Autodesk Inventor part; units mm, degrees
ref_plane "YZ Plane" through (0, 0, 0) normal (1, 0, 0) x (0, 1, 0)
ref_plane "XZ Plane" through (0, 0, 0) normal (0, 1, 0) x (-1, 0, 0)
ref_plane "XY Plane" through (0, 0, 0) normal (0, 0, 1) x (1, 0, 0)
sketch "Sketch1" plane through (0, 0, 0) normal (0, 0, 1) x (1, 0, 0)
  line L0 (0, 0) -> (150, 0)
  line L1 (150, 0) -> (150, -135)
  line L2 (150, -135) -> (0, -135)
  line L3 (0, -135) -> (0, 0)
  circle A0 centre (3.5, -35) radius 1.5
  line L4 (75, 0) -> (75, -135)
  circle A1 centre (146.5, -35) radius 1.5
  circle A2 centre (3.5, -125) radius 1.5
  circle A3 centre (146.5, -125) radius 1.5
  dimension "d0" = 150
  dimension "d1" = 135
  dimension "d2" = 3
  dimension "d3" = 3.5
  dimension "d4" = 35
  dimension "d5" = 3
  dimension "d6" = 3.5
  dimension "d7" = 90
extrude "Extrusion1" add sketch "Sketch1" along normal blind 7
move faces "Move1" translate (0, -0.3, 0) faces at (100, 0, 2.3333)
move faces "Move2" translate (-0.3, 0, 0) faces at (150, -90.1, 2.3333)
move faces "Move3" translate (0, 0.3, 0) faces at (49.9, -135, 2.3333)
move faces "Move4" translate (0.3, 0, 0) faces at (0, -45.1, 2.3333)
sketch "Sketch3" plane through (0, 0, 0) normal (0, 0, -1) x (-1, 0, 0)
  line L0 (-149.7, -134.7) -> (-149.7, -0.3) construction
  line L1 (-149.7, -23.3) -> (-0.3, -23.3) construction
  line L2 (-0.3, -0.3) -> (-0.3, -134.7) construction
  line L3 (-149.7, -0.3) -> (-0.3, -0.3) construction
  line L4 (-125, -28.3) -> (-25, -28.3)
  line L5 (-25, -28.3) -> (-25, -18.3)
  line L6 (-25, -18.3) -> (-125, -18.3)
  line L7 (-125, -18.3) -> (-125, -28.3)
  line L8 (-125, -28.3) -> (-25, -18.3) construction
  line L9 (-25, -28.3) -> (-125, -18.3) construction
  line L10 (-149.7, -0.3) -> (-0.3, -0.3)
  line L11 (-75, -0.3) -> (-75, -132.391)
  circle A0 centre (-112.5, -69.7) radius 2.5
  line L12 (-0.3, -134.7) -> (-149.7, -134.7)
  circle A1 centre (-37.5, -69.7) radius 2.5
  point P0 (0, 0)
  point P1 (-75, -23.3)
  dimension "d22" = 23
  dimension "d23" = 100
  dimension "d24" = 10
  dimension "d27" = 5
  dimension "d28" = 75
  dimension "d29" = 65
extrude "Extrusion2" cut sketch "Sketch3" against normal through all
sketch "Sketch5" plane through (0, 0, 7) normal (0, 0, 1) x (1, 0, 0)
  point P0 (0, 0)
sketch "Sketch6" plane through (0.3, -134.7, 0) normal (-1, 0, 0) x (0, 0, 1)
  point P0 (0, 134.7)
properties part number "mávač_víčko"
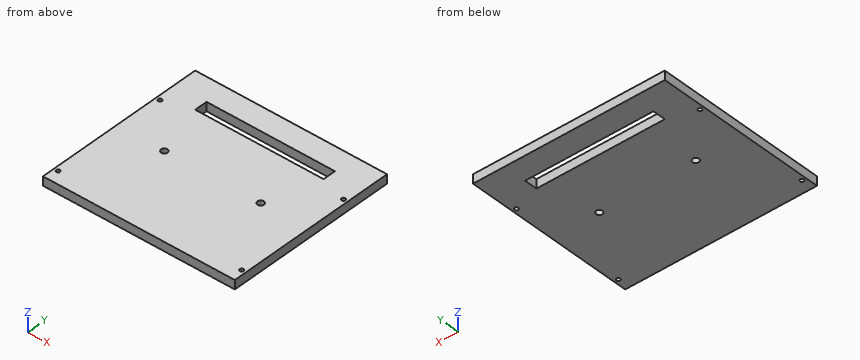
The listing builds one solid part. Answer for the finished solid, in the listing's coordinates (mm). Coordinates: 2 decimals unless noted, no trailing zeros. Loops run counter-clockwise (first coordinate to the right, second up) from the corner with the lowest first, then second, coordinate; pieces in that order, holes last.
1) Find section A-A on x = 112.5. Write down the section's boundary in (y, z), then the cut area to 3 significant figures.
2) Find section C-C on x = 94.5. Write down the section's boundary in (y, z), then the cut area to 3 significant figures.
3) A flat-ended cylindrical pin translates along its axis: pin 1 Ø5 at (x, y) = (146.5, -125) entering from +Z. Find the tip coordinate at first contact, or state that the pin passes through.
4) Find the intervals of material crossed by L1, parallel to X at y = -125, z = 3.25; L2, parallel to Y at x = 37.5, z = 2.75; L3, parallel to Y at x = 146.5, z = 5, in increasing order.
5) Find section B-B on z = 3.5. Write down the section's boundary in (x, y).
Values:
1. outline: (-134.7, 0) - (-72.2, 0) - (-72.2, 7) - (-134.7, 7) - close; (-67.2, 0) - (-28.3, 0) - (-28.3, 7) - (-67.2, 7) - close; (-18.3, 0) - (-0.3, 0) - (-0.3, 7) - (-18.3, 7) - close
1. area: 836 mm2
2. outline: (-134.7, 0) - (-28.3, 0) - (-28.3, 7) - (-134.7, 7) - close; (-18.3, 0) - (-0.3, 0) - (-0.3, 7) - (-18.3, 7) - close
2. area: 871 mm2
3. pin 1: stops at z = 7
4. L1: x = 0.3 to 2, 5 to 145, 148 to 149.7
4. L2: y = -134.7 to -72.2, -67.2 to -28.3, -18.3 to -0.3
4. L3: y = -134.7 to -126.5, -123.5 to -36.5, -33.5 to -0.3
5. outline: (0.3, -134.7) - (149.7, -134.7) - (149.7, -0.3) - (0.3, -0.3) - close; hole circle Ø3 at (3.5, -125); hole circle Ø3 at (3.5, -35); hole (25, -28.3) - (125, -28.3) - (125, -18.3) - (25, -18.3) - close; hole circle Ø5 at (37.5, -69.7); hole circle Ø5 at (112.5, -69.7); hole circle Ø3 at (146.5, -125); hole circle Ø3 at (146.5, -35)
